Autodesk Inventor part; units mm, degrees
ref_plane "YZ Plane" through (0, 0, 0) normal (1, 0, 0) x (0, 1, 0)
ref_plane "XZ Plane" through (0, 0, 0) normal (0, 1, 0) x (-1, 0, 0)
ref_plane "XY Plane" through (0, 0, 0) normal (0, 0, 1) x (1, 0, 0)
sketch "Sketch1" plane through (0, 0, 0) normal (0, 1, 0) x (-1, 0, 0)
  line L0 (-16, 12.5) -> (-16, -12.5)
  line L1 (16, 12.5) -> (-16, 12.5)
  line L2 (16, -12.5) -> (16, 12.5)
  line L3 (-16, -12.5) -> (16, -12.5)
extrude "Extrusion1" add sketch "Sketch1" along normal blind 6
hole "Hole5" at (0, 6, 0) direction (0, -1, 0) diameter 10 depth 6
hole "Hole4" at (-11, 6, -7.5) direction (0, -1, 0) diameter 4.5 depth 6
sketch "Sketch4" plane through (0, 6, 0) normal (0, 1, 0) x (1, 0, 0)
  point P0 (11, -7.5)
hole "Hole3" at (11, 6, 7.5) direction (0, -1, 0) diameter 4.5 depth 6
sketch "Sketch3" plane through (0, 6, 0) normal (0, 1, 0) x (1, 0, 0)
  point P0 (-11, 7.5)
hole "Hole2" at (11, 6, -7.5) direction (0, -1, 0) diameter 4.5 depth 6
sketch "Sketch2" plane through (0, 6, 0) normal (0, 1, 0) x (1, 0, 0)
  point P0 (0, 0)
hole "Hole1" at (-11, 6, 7.5) direction (0, -1, 0) diameter 4.5 depth 6
sketch "Sketch5" plane through (0, 6, 0) normal (0, 1, 0) x (1, 0, 0)
  point P0 (11, 7.5)
sketch "Sketch6" plane through (0, 6, 0) normal (0, 1, 0) x (1, 0, 0)
  point P0 (-11, -7.5)
properties part number "Hopper Nut Trap Holder" material "ASA Plastic"
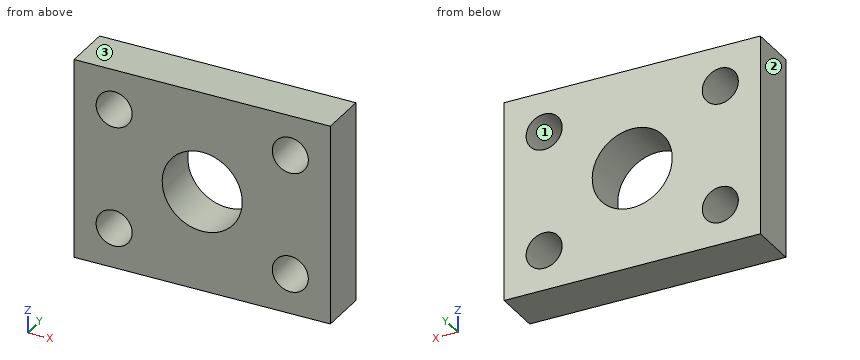
Geometry check sheet. Reference: the model listing, model coordinates, mm. Face numbers are marked on the shaded views. Round coordinates to 2 decimals unless told otherwise and drop trailing zeros. Write each loop counter-clockwise with the first axis right and the second up, starting at its lowest first coordinate (ties: lowest second). Pieces come first, ordered by that corner, then holes.
Item 1: Section check C-C (x = 0). Record the boundary of the cut face in (y, z), plus the area to 3 significant figures.
Determined:
outline: (0, -12.5) - (6, -12.5) - (6, -5) - (0, -5) - close; (0, 5) - (6, 5) - (6, 12.5) - (0, 12.5) - close
area: 90.0 mm2
Item 2: Mould release check, pull along Z, two halves, no side actions. Record for the marked faces 1, 2 and 3: +Z half, -Z half, draft (parallel to the pull), parting line (faces both ways), or undercut.
Determined:
face 1: undercut
face 2: draft
face 3: +Z half
Item 3: Material ranges on line 1 along X through (y, z) = (3.55, 7.5); line 2 along Z through (x, y) = (11, 2.4); line 3 along X through (y, z) = (1.8, 0), recorded low to high.
Determined:
line 1: x = -16 to -13.25, -8.75 to 8.75, 13.25 to 16
line 2: z = -12.5 to -9.75, -5.25 to 5.25, 9.75 to 12.5
line 3: x = -16 to -5, 5 to 16
Item 4: Section check A-A (x = -11). Record the boundary of the cut face in (y, z).
Determined:
outline: (0, -12.5) - (6, -12.5) - (6, -9.75) - (0, -9.75) - close; (0, -5.25) - (6, -5.25) - (6, 5.25) - (0, 5.25) - close; (0, 9.75) - (6, 9.75) - (6, 12.5) - (0, 12.5) - close
Item 5: Section check B-B (z = -7.5). Record the boundary of the cut face in (x, y), plus the area to 3 significant figures.
Determined:
outline: (-16, 0) - (-13.25, 0) - (-13.25, 6) - (-16, 6) - close; (-8.75, 0) - (8.75, 0) - (8.75, 6) - (-8.75, 6) - close; (13.25, 0) - (16, 0) - (16, 6) - (13.25, 6) - close
area: 138 mm2
Item 6: Section check D-D (y = 3.05). Record the boundary of the cut face in (x, z), plus the area to 3 significant figures.
Determined:
outline: (-16, -12.5) - (16, -12.5) - (16, 12.5) - (-16, 12.5) - close; hole circle Ø4.5 at (-11, -7.5); hole circle Ø4.5 at (-11, 7.5); hole circle Ø10 at (0, 0); hole circle Ø4.5 at (11, -7.5); hole circle Ø4.5 at (11, 7.5)
area: 658 mm2
